The listing builds one solid part. Answer for the finished solid, in the listing's coordinates (mm). Face numbers are marked on the shaded views. A direction names the side the tool comes from. Coordinates: 2 decimals unless noted, no trailing zeros. Write each loop counter-clockwise with the first axis right and the second up, starting at its lowest first coordinate (ties: lowest second). Pieces come first, ordered by that corner, then holes.
from build123d import *

# Parameters (mm, degrees)
LINEAR_AUSTRAGEN_D_NN1_DEPTH    = 30
FASE1_SIZE                      = 1
SKIZZE2_R                       = 1.5
SCHNITT_LINEAR_AUSTRAGEN1_DEPTH = 10
SKIZZE3_R                       = 1.5
SCHNITT_LINEAR_AUSTRAGEN2_DEPTH = 10


with BuildPart() as part:
    # Skizze1 → Linear-Austragen-Dünn1 (new, symmetric)
    with BuildSketch(Plane.XY):
        Polygon((0, 10), (0, 0), (10, 0), (10, 1), (1, 1), (1, 10), align=None)
    extrude(amount=LINEAR_AUSTRAGEN_D_NN1_DEPTH, both=True)

    # Fase1
    fase1_edges = [part.edges().sort_by_distance(p)[0] for p in [
        (0.5, 10, 30),
        (0.5, 10, -30),
        (10, 0.5, -30),
        (10, 0.5, 30),
    ]]
    chamfer(fase1_edges, length=FASE1_SIZE)

    # Skizze2 → Schnitt-Linear austragen1 (cut)
    with BuildSketch(Plane(origin=(1, 0, 0), x_dir=(0, 0, -1), z_dir=(1, 0, 0))):
        with Locations(Location((-15, 6, 0), (0, 0, 90))):
            Circle(SKIZZE2_R)
        with Locations(Location((15, 6, 0), (0, 0, 90))):
            Circle(SKIZZE2_R)
        with Locations(Location((-25, 6, 0), (0, 0, 90))):
            Circle(SKIZZE2_R)
        with Locations(Location((25, 6, 0), (0, 0, 90))):
            Circle(SKIZZE2_R)
    extrude(amount=-SCHNITT_LINEAR_AUSTRAGEN1_DEPTH, mode=Mode.SUBTRACT)

    # Skizze3 → Schnitt-Linear austragen2 (cut)
    with BuildSketch(Plane(origin=(0, 1, 0), x_dir=(1, 0, 0), z_dir=(0, 1, 0))):
        with Locations(Location((6, -20, 0), (0, 0, 270))):
            Circle(SKIZZE3_R)
        with Locations(Location((6, 20, 0), (0, 0, 270))):
            Circle(SKIZZE3_R)
    extrude(amount=-SCHNITT_LINEAR_AUSTRAGEN2_DEPTH, mode=Mode.SUBTRACT)


solid = part.part
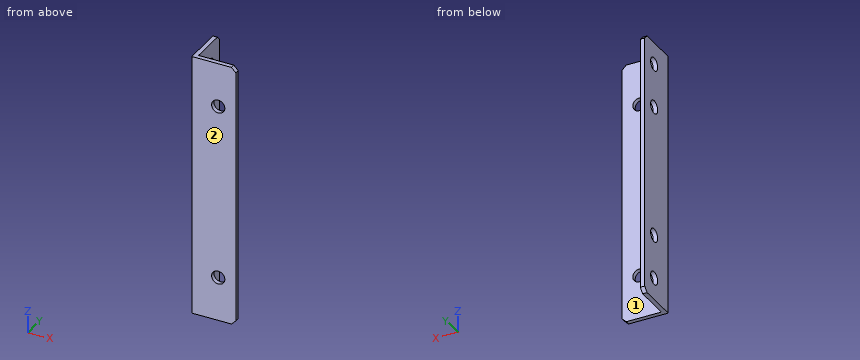
Q1. The part is cut by section B-B, the plane x = 6. Write down the section's boundary in (y, z).
Answers below:
outline: (0, -30) - (1, -30) - (1, -21.5) - (0, -21.5) - close; (0, -18.5) - (1, -18.5) - (1, 18.5) - (0, 18.5) - close; (0, 21.5) - (1, 21.5) - (1, 30) - (0, 30) - close
Q2. The part is cut by section A-A, the plane z = 25. Write down the section's boundary in (x, y).
Answers below:
outline: (0, 0) - (10, 0) - (10, 1) - (1, 1) - (1, 4.5) - (0, 4.5) - close; (0, 7.5) - (1, 7.5) - (1, 10) - (0, 10) - close
Q3. The part is cut by section C-C, the plane y = 6. Write down the section's boundary in (x, z), then the cut area to 3 significant figures.
Answers below:
outline: (0, -30) - (1, -30) - (1, -26.5) - (0, -26.5) - close; (0, -23.5) - (1, -23.5) - (1, -16.5) - (0, -16.5) - close; (0, -13.5) - (1, -13.5) - (1, 13.5) - (0, 13.5) - close; (0, 16.5) - (1, 16.5) - (1, 23.5) - (0, 23.5) - close; (0, 26.5) - (1, 26.5) - (1, 30) - (0, 30) - close
area: 48.0 mm2
Q4. Given pin 1 (2.5 mm diameter, centred on y = 7, z = 8, fed in from +X); pin 2 (2.5 mm diameter, centred on y = 6, z = 25, fed in from -X); pin 3 (1 mm diameter, centred on x = 5.5, z = 10, fed in from +Y), each flat-ended and moving along its own axis, determine where each tip first touches the part or whether it passes through.
Answers below:
pin 1: stops at x = 1
pin 2: passes through
pin 3: stops at y = 1
Q5. The part is cut by section D-D, the plane z = -12.5. Write down the section's boundary in (x, y), then the cut area to 3 significant figures.
Answers below:
outline: (0, 0) - (10, 0) - (10, 1) - (1, 1) - (1, 10) - (0, 10) - close
area: 19.0 mm2
Q6. Find the intervals of material crossed by probe 1 along Z at (x, y) = (0.75, 6); probe 2 along X at (y, z) = (0.65, -20); probe 3 along Y at (x, z) = (2.5, 1), in increasing order.
Answers below:
probe 1: z = -30 to -26.5, -23.5 to -16.5, -13.5 to 13.5, 16.5 to 23.5, 26.5 to 30
probe 2: x = 0 to 4.5, 7.5 to 10
probe 3: y = 0 to 1
Q7. Which of the six approach directions +Z, -Z, +X, -X, +Y, -Y give full straight-line access (tool end or side, diameter ignored) to the marked faces 1 and 2?
Answers below:
face 1: +Z, -Z, +X, +Y
face 2: +Z, -Z, +X, -X, -Y
